Design review of the part built by this model. Coordinates are the model's own, in mm. Face numbers are marked on the shaded views. Give positions to 0.01 mm unless a question says otherwise; leave off trailing zeros. Write each loop counter-clockwise with the first axis right and the second up, starting at its lowest first coordinate (ties: lowest second). Pieces come first, ordered by that corner, then holes. Notation, with made-up numbers: (7, -21) -> (37, -21) arc R36 cw to (37, 18) -> close; hole circle Ø1 at (-23, 4). An arc over 180 degrees is marked (long way). Write each question's results on one line, items separated by ' | '. Start each with the question number.
(1) Mouldability with a two-part tool opening along Y and no side actions: class the marked faces 1 and 2 as released by +Y, released by -Y, zero draft, split by the parting line, or undercut.
(2) Clearance check with flat-ended pins moving along their axes: pin 1 (8 mm diameter, centred on x = 65, y = 75, fed in from +Z); pin 2 (20.5 mm diameter, centred on x = 76.2, y = 406.4, fed in from +Z); pin 3 (20.5 mm diameter, centred on x = 76.2, z = 0, fed in from +Y); pin 4 (14 mm diameter, centred on y = 0, z = 0, fed in from +X). State where each tip first meets the part, or that it passes through.
(3) Take a section at A-A (y = 342). State the section outline as (x, z) points (3 decimals).
(4) To check wall thickness, follow probe 1 along Z at (x, y) = (19, 0) (3 decimals); probe 2 along Y at (x, z) = (76, 44); probe 3 along X at (y, z) = (201.5, 0) (3 decimals). State the ranges of each line that lie inside material, in increasing order.
(5) Take a section at B-B (x = 8.5). State the section outline as (y, z) points (3 decimals), plus the area to 3 significant figures.
from build123d import *

# Parameters (mm, degrees)
SKETCH1_R            = 9.525
SKETCH1_R_2          = 7.874
SWEEP2_START         = 25.3999999
SWEEP2_OUTLINE_R     = 9.525
SWEEP2_OUTLINE_R_2   = 7.874
SWEEP2_DEPTH         = 50.8000001
SWEEP2_2_OUTLINE_R   = 9.525
SWEEP2_2_OUTLINE_R_2 = 7.874
SWEEP2_2_ANGLE       = 90


with BuildPart() as part:
    # Sweep1: sweep along a path in Sketch2
    with BuildLine(Plane.XY) as sweep1_path:
        Line((76.2, 381), (76.2, 25.4))
        ThreePointArc((76.2, 25.4), (68.760512242, 7.439487758), (50.8, 0))
        Line((50.8, 0), (0, 0))
    # Sketch1 → Sweep1 (sweep)
    with BuildSketch(Plane(origin=(0, 0, 0), x_dir=(0, -1, 0), z_dir=(1, 0, 0))):
        Circle(SKETCH1_R)
        Circle(SKETCH1_R_2, mode=Mode.SUBTRACT)
    sweep(path=sweep1_path.line)



with BuildPart() as body_2:
    # Sweep2: read off the stored shape, not the designer's step
    # Sweep2 outline → Sweep2 (new body)
    with BuildSketch(Plane.XY.offset(SWEEP2_START)):
        with Locations((76.2, 406.4)):
            Circle(SWEEP2_OUTLINE_R)
        with Locations((76.2, 406.4)):
            Circle(SWEEP2_OUTLINE_R_2, mode=Mode.SUBTRACT)
    extrude(amount=SWEEP2_DEPTH)


with BuildPart() as part_1:
    add(part.part)

    add(body_2.part)  # Sweep2 2 merges body 2
    # Sweep2 2 outline → Sweep2 2 (revolve)
    with BuildSketch(Plane(origin=(0, 381, 25.4), x_dir=(0, 0, -1), z_dir=(0, -1, 0))):
        with Locations((25.4, 76.2)):
            Circle(SWEEP2_2_OUTLINE_R)
        with Locations((25.4, 76.2)):
            Circle(SWEEP2_2_OUTLINE_R_2, mode=Mode.SUBTRACT)
    revolve(axis=Axis((0, 381, 25.4), (1, 0, 0)), revolution_arc=SWEEP2_2_ANGLE)


solid = part_1.part
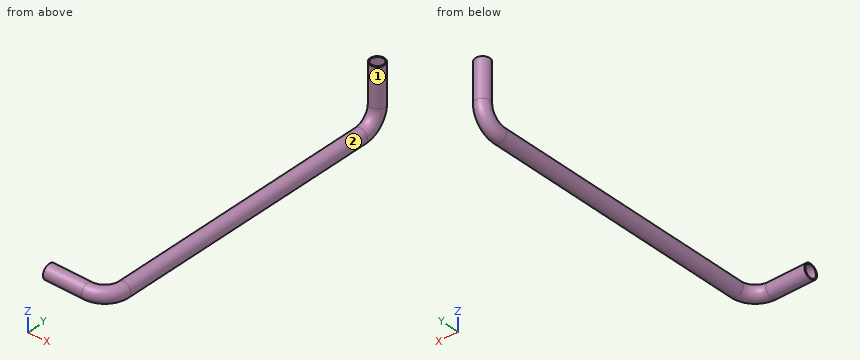
Report:
1) face 1: split by the parting line | face 2: undercut
2) pin 1: z = 6.24 | pin 2: z = 76.2 | pin 3: y = 412.47 | pin 4: x = 80.48
3) outline: circle Ø19.05 at (76.2, 0); hole circle Ø15.748 at (76.2, 0)
4) probe 1: -9.525 to -7.874, 7.874 to 9.525 | probe 2: 396.88 to 398.53, 414.27 to 415.92 | probe 3: 66.675 to 68.326, 84.074 to 85.725
5) outline: circle Ø19.05 at (0, 0); hole circle Ø15.748 at (0, 0) | area: 90.2 mm2
